Could you check a few things on this model? Use its own coordinates, in mm. Coordinates: 2 decimals unless noted, no trailing zeros. Write each loop counter-clockwise with the first axis right and the second up, starting at its lowest first coordinate (ties: lowest second). Pieces come first, ordered by that corner, then holes.
Item 1: I want a section at C-C on z = 0. Please give me the cut outline in (x, y).
Item 2: I want a section at B-B on z = -150. Please give me the cut outline in (x, y).
Item 3: I want a section at A-A on x = 150. Please give me the cut outline in (y, z), then the cut area to 4 significant figures.
Item 4: I want a section at D-D on y = 3.5. Please give me the cut outline in (x, z), then the cut area to 3 significant figures.
Item 5: If I drill on probe 1 along X at (y, z) = (7.25, 0); probe 2 along X at (y, z) = (3, -150); probe 3 along X at (y, z) = (0.5, 12), over which ranges is the centre line in solid material (lowest first)?
Item 6: For P1, Ø1, axis at x = 12, z = 73.5, coming from the -Y side; P2, Ø5, axis at y = 4, z = -99.5, coming from the +X side; P3, Ø5, axis at x = 57.5, y = 5, coming from the +Z side; P4, Ø4, axis at y = 1.5, z = -92.5, coming from the -X side, each with a flat end and sliding along its axis, tell me the tip position at first contact or that it passes through.
from build123d import *

# Parameters (mm, degrees)
SKETCH1_R           = 15
SKETCH1_W           = 30
SKETCH1_H           = 30
BOSS_EXTRUDE2_DEPTH = 10


with BuildPart() as part:
    # Sketch1 → Boss-Extrude2 (new body)
    # profile 1 of 5: a face of its own
    with BuildSketch(Plane(origin=(0, 0, 0), x_dir=(1, 0, 0), z_dir=(0, 1, 0))):
        with BuildLine():
            Line((15, -15), (-15, -15))
            Line((-15, -15), (-15, -136.771243445))
            ThreePointArc((-15, -136.771243445), (0, -170), (15, -136.771243445))
            Line((15, -136.771243445), (15, -15))
        make_face()
        with Locations(Location((0, -150, 0), (0, 0, 270))):
            Circle(SKETCH1_R, mode=Mode.SUBTRACT)
    # profile 2 of 5: a face of its own
    with BuildSketch(Plane(origin=(0, 0, 0), x_dir=(1, 0, 0), z_dir=(0, 1, 0))):
        Rectangle(SKETCH1_W, SKETCH1_H)
    # profile 3 of 5: a face of its own
    with BuildSketch(Plane(origin=(0, 0, 0), x_dir=(1, 0, 0), z_dir=(0, 1, 0))):
        with BuildLine():
            Line((-15, 136.771243445), (-15, 15))
            Line((-15, 15), (15, 15))
            Line((15, 15), (15, 136.771243445))
            ThreePointArc((15, 136.771243445), (0, 170), (-15, 136.771243445))
        make_face()
        with Locations(Location((0, 150, 0), (0, 0, 270))):
            Circle(SKETCH1_R, mode=Mode.SUBTRACT)
    # profile 4 of 5: a face of its own
    with BuildSketch(Plane(origin=(0, 0, 0), x_dir=(1, 0, 0), z_dir=(0, 1, 0))):
        with BuildLine():
            Line((-15, 15), (-136.771243445, 15))
            ThreePointArc((-136.771243445, 15), (-170, 0), (-136.771243445, -15))
            Line((-136.771243445, -15), (-15, -15))
            Line((-15, -15), (-15, 15))
        make_face()
        with Locations(Location((-150, 0, 0), (0, 0, 270))):
            Circle(SKETCH1_R, mode=Mode.SUBTRACT)
    # profile 5 of 5: a face of its own
    with BuildSketch(Plane(origin=(0, 0, 0), x_dir=(1, 0, 0), z_dir=(0, 1, 0))):
        with BuildLine():
            Line((136.771243445, 15), (15, 15))
            Line((15, 15), (15, -15))
            Line((15, -15), (136.771243445, -15))
            ThreePointArc((136.771243445, -15), (170, 0), (136.771243445, 15))
        make_face()
        with Locations(Location((150, 0, 0), (0, 0, 270))):
            Circle(SKETCH1_R, mode=Mode.SUBTRACT)
    extrude(amount=BOSS_EXTRUDE2_DEPTH)


solid = part.part
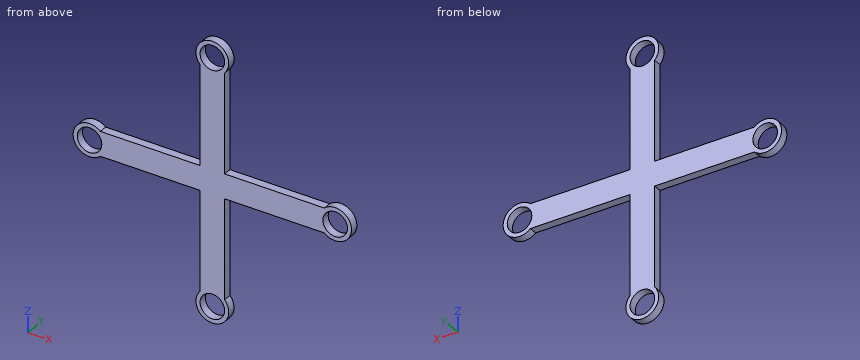
Response values:
1. outline: (-170, 0) - (-165, 0) - (-165, 10) - (-170, 10) - close; (-135, 0) - (135, 0) - (135, 10) - (-135, 10) - close; (165, 0) - (170, 0) - (170, 10) - (165, 10) - close
2. outline: (-20, 0) - (-15, 0) - (-15, 10) - (-20, 10) - close; (15, 0) - (20, 0) - (20, 10) - (15, 10) - close
3. outline: (0, -20) - (10, -20) - (10, -15) - (0, -15) - close; (0, 15) - (10, 15) - (10, 20) - (0, 20) - close
3. area: 100.0 mm2
4. outline: (-136.77, -15) - (-15, -15) - (-15, -136.77) arc R20 ccw (long way) to (15, -136.77) - (15, -15) - (136.77, -15) arc R20 ccw (long way) to (136.77, 15) - (15, 15) - (15, 136.77) arc R20 ccw (long way) to (-15, 136.77) - (-15, 15) - (-136.77, 15) arc R20 ccw (long way) to start; hole circle Ø30 at (-150, 0); hole circle Ø30 at (0, -150); hole circle Ø30 at (0, 150); hole circle Ø30 at (150, 0)
4. area: 17,100 mm2
5. probe 1: x = -170 to -165, -135 to 135, 165 to 170
5. probe 2: x = -20 to -15, 15 to 20
5. probe 3: x = -166 to -159, -141 to 141, 159 to 166
6. P1: stops at y = 0
6. P2: stops at x = 15
6. P3: stops at z = 15
6. P4: stops at x = -15
